from build123d import *

# Parameters (mm, degrees)
SKETCH3_W               = 47.4
SKETCH3_H               = 42.1
BOSS_EXTRUDE1_DEPTH     = 2
SKETCH4_W               = 2.2
SKETCH4_H               = 5
BOSS_EXTRUDE2_DEPTH     = 8
SKETCH6_W               = 2.2
SKETCH6_H               = 2
BOSS_EXTRUDE3_DEPTH     = 9.8
BOSS_EXTRUDE5_REACH     = 57.631
SKETCH10_W              = 9.8
SKETCH10_H              = 2
MIRROR3_COPY_1_SKETCH_W = 2.2
MIRROR3_COPY_1_SKETCH_H = 5
MIRROR3_COPY_1_DEPTH    = 8
MIRROR3_COPY_2_SKETCH_W = 2.2
MIRROR3_COPY_2_SKETCH_H = 2
MIRROR3_COPY_2_DEPTH    = 9.8
SKETCH7_W               = 25
SKETCH7_H               = 25
CUT_EXTRUDE1_DEPTH      = 2


with BuildPart() as part:
    # Sketch3 → Boss-Extrude1 (new body)
    with BuildSketch(Plane(origin=(0, 0, 0), x_dir=(1, 0, 0), z_dir=(0, 1, 0))):
        Rectangle(SKETCH3_W, SKETCH3_H)
    extrude(amount=BOSS_EXTRUDE1_DEPTH)

    # Sketch4 → Boss-Extrude2 (add)
    with BuildSketch(Plane(origin=(0, 2, 0), x_dir=(1, 0, 0), z_dir=(0, 1, 0))):
        with Locations((-22.6, 18.55)):
            Rectangle(SKETCH4_W, SKETCH4_H)
    boss_extrude2 = extrude(amount=BOSS_EXTRUDE2_DEPTH)

    # Sketch6 → Boss-Extrude3 (add)
    with BuildSketch(Plane(origin=(0, 0, -21.05), x_dir=(-1, 0, 0), z_dir=(0, 0, -1))):
        with Locations((22.6, 9)):
            Rectangle(SKETCH6_W, SKETCH6_H)
    boss_extrude3 = extrude(amount=BOSS_EXTRUDE3_DEPTH)

    # Mirror1: Boss-Extrude2, Boss-Extrude3 across plane
    add(boss_extrude2.mirror(Plane(origin=(0, 0, 0), x_dir=(0, 0, 1), z_dir=(1, 0, 0))))
    add(boss_extrude3.mirror(Plane(origin=(0, 0, 0), x_dir=(0, 0, 1), z_dir=(1, 0, 0))))

    # Sketch10 → Boss-Extrude5 (add, up to next)
    with BuildSketch(Plane(origin=(-21.5, 0, 0), x_dir=(0, 0, -1), z_dir=(1, 0, 0)), mode=Mode.PRIVATE) as boss_extrude5_sk1:
        with Locations((25.95, 9)):
            Rectangle(SKETCH10_W, SKETCH10_H)
    boss_extrude5_tool1 = extrude(boss_extrude5_sk1.sketch, amount=BOSS_EXTRUDE5_REACH, mode=Mode.PRIVATE) - part.part
    boss_extrude5 = boss_extrude5_tool1.solids().sort_by_distance((-21.5, 9, -25.95))[0]
    add(boss_extrude5)

    # Mirror3: Boss-Extrude2, Boss-Extrude3, Boss-Extrude5 across plane
    add(boss_extrude2.mirror(Plane.XY))
    add(boss_extrude3.mirror(Plane.XY))
    add(boss_extrude5.mirror(Plane.XY))

    # Mirror3 copy 1 sketch → Mirror3 copy 1 (add)
    with BuildSketch(Plane(origin=(0, 2, 0), x_dir=(-1, 0, 0), z_dir=(0, 1, 0))):
        with Locations((-22.6, 18.55)):
            Rectangle(MIRROR3_COPY_1_SKETCH_W, MIRROR3_COPY_1_SKETCH_H)
    extrude(amount=MIRROR3_COPY_1_DEPTH)

    # Mirror3 copy 2 sketch → Mirror3 copy 2 (add)
    with BuildSketch(Plane.XY.offset(21.05)):
        with Locations((22.6, 9)):
            Rectangle(MIRROR3_COPY_2_SKETCH_W, MIRROR3_COPY_2_SKETCH_H)
    extrude(amount=MIRROR3_COPY_2_DEPTH)

    # Sketch7 → Cut-Extrude1 (cut)
    with BuildSketch(Plane.XZ):
        Rectangle(SKETCH7_W, SKETCH7_H)
    extrude(amount=-CUT_EXTRUDE1_DEPTH, mode=Mode.SUBTRACT)


solid = part.part
Check sheet for the modelled part. Datum: model origin and axes. Units: mm. A direction names the side the tool comes from. Round coordinates to 2 decimals unless told otherwise and drop trailing zeros. Loops run counter-clockwise (first coordinate to the right, second up) from the corner with the lowest first, then second, coordinate; pieces in that order, holes last.
1. Scan lines: probe 1 along Z at (x, y) = (-5.5, 8.75); probe 2 along Y at (x, z) = (-1, 21); probe 3 along Z at (x, y) = (-2.5, 1). Record each from-to range of solid material in increasing order.
2. Gauge pin test, flat ends, axial feed: pin 1 Ø2.5 at (x, y) = (-22.5, 5) entering from +Z; pin 2 Ø5 at (x, z) = (-4.5, -25) entering from -Y; pin 3 Ø1.1 at (x, y) = (22.5, 4) entering from -Z; pin 4 Ø10 at (x, z) = (1, 3) entering from +Y. Record the tip position at first contact, or that the pin passes through.
3. Mould release check, pull along X, two halves, no side actions. Record for faces 1 (the flat face through (-23.7, 1.6, -0.4)), 2 (the flat face through (21.5, 6, -19)), 3 (the flat face through (23, 6, -16.05)): released by +X, released by -X, zero draft, split by the parting line, or undercut.
4. Sectioned sample at D-D on y = 9.25. Record the boundary of the cut face in (x, z).
5. Sectioned sample at C-C on x = 10.5. Record the boundary of the cut face in (y, z).
6. Set-up check for faces 4 (the flat face through (-21.5, 6, -19)), 5 (the flat face through (23, 6, 16.05)), 6 (the flat face through (-12.5, 1, 0)): record each of +Z, -Z, +X, -X, +Y, -Y from which the full face is reachable in a straight line by a thin tool's end or side.
7. Sectioned sample at A-A on y = 6.25. Record the boundary of the cut face in (x, z).
8. Sectioned sample at B-B on z = 1. Record the boundary of the cut face in (x, y), and give its area (3 significant figures).
Recorded:
1. probe 1: z = -30.85 to -21.05, 21.05 to 30.85
1. probe 2: y = 0 to 2
1. probe 3: z = -21.05 to -12.5, 12.5 to 21.05
2. pin 1: stops at z = 21.05
2. pin 2: stops at y = 8
2. pin 3: stops at z = -21.05
2. pin 4: passes through
3. face 1: released by -X
3. face 2: undercut
3. face 3: zero draft
4. outline: (-23.7, -30.85) - (23.7, -30.85) - (23.7, -16.05) - (21.5, -16.05) - (21.5, -21.05) - (-21.5, -21.05) - (-21.5, -16.05) - (-23.7, -16.05) - close; (-23.7, 16.05) - (-21.5, 16.05) - (-21.5, 21.05) - (21.5, 21.05) - (21.5, 16.05) - (23.7, 16.05) - (23.7, 30.85) - (-23.7, 30.85) - close
5. outline: (0, -21.05) - (2, -21.05) - (2, -12.5) - (0, -12.5) - close; (0, 12.5) - (2, 12.5) - (2, 21.05) - (0, 21.05) - close; (8, -30.85) - (10, -30.85) - (10, -21.05) - (8, -21.05) - close; (8, 21.05) - (10, 21.05) - (10, 30.85) - (8, 30.85) - close
6. face 4: +Y
6. face 5: +X, -X, +Y
6. face 6: +Y, -Y
7. outline: (-23.7, -21.05) - (-21.5, -21.05) - (-21.5, -16.05) - (-23.7, -16.05) - close; (-23.7, 16.05) - (-21.5, 16.05) - (-21.5, 21.05) - (-23.7, 21.05) - close; (21.5, -21.05) - (23.7, -21.05) - (23.7, -16.05) - (21.5, -16.05) - close; (21.5, 16.05) - (23.7, 16.05) - (23.7, 21.05) - (21.5, 21.05) - close
8. outline: (-23.7, 0) - (-12.5, 0) - (-12.5, 2) - (-23.7, 2) - close; (12.5, 0) - (23.7, 0) - (23.7, 2) - (12.5, 2) - close
8. area: 44.8 mm2
